Input: part model. Units: mm. Frame: model coordinates. A direction names the side the tool comes from. Round coordinates to 2 decimals unless told otherwise and drop trailing zeros. Loops run counter-clockwise (first coordinate to the right, second up) from the corner with the lowest first, then second, coordinate; pieces in that order, holes last. Notation, with made-up numbers: (32, 60.25) -> (44, 60.25) arc R21 ccw to (44, 69.25) -> close; hole circle Ø8 at (-21.5, 31.25). An arc over 180 degrees is marked (long way). Answer as a JSON object with one key per item and string values. Group by question number.
Item 1: Section query B-B on y = 15. Return loops of the section in (x, z) (3 decimals), and give its area (3 significant figures).
Item 2: Set-up query: faces 1 (the flat face through (6.35, 12, 2)), 2 (the flat face through (6, 3, -107.95)). Return all of +Z, -Z, +X, -X, +Y, -Y with unobstructed straight access to the full face (end or side cutting, diameter ignored); none if empty.
Item 3: Pin query (flat end, axial travel): pin 1 (2.5 mm diameter, centred on x = -0.29, z = -95.25, fed in from +Y); pin 2 (4.5 mm diameter, centred on x = -0.29, z = 95.25, fed in from +Y) (3 decimals); pin 3 (10 mm diameter, centred on y = 14.5, z = 49, fed in from -X). Return the tip coordinate at first contact, or that it passes through.
Item 4: Material intervals for line 1 (X direction, y = 1.5, z = -95.25) (3 decimals); line 2 (Y direction, x = -0.5, z = -71.5) (3 decimals); line 3 (X direction, y = 6.5, z = -58.5) (3 decimals), sorted ascending. Write a range as [from, to].
from build123d import *

# Parameters (mm, degrees)
BOSS_EXTRUDE1_DEPTH   = 107.95
F_6_32_TAPPED_HOLE1_D = 2.7051


with BuildPart() as part:
    # Sketch2 → Boss-Extrude1 (new, symmetric)
    with BuildSketch(Plane.XY):
        with BuildLine():
            Line((-9.525, 0), (9.525, 0))
            Line((9.525, 0), (9.525, 19.05))
            Line((9.525, 19.05), (7.9375, 19.05))
            ThreePointArc((7.9375, 19.05), (6.814967985, 18.585032015), (6.35, 17.4625))
            Line((6.35, 17.4625), (6.35, 6.35))
            ThreePointArc((6.35, 6.35), (5.42006403, 4.10493597), (3.175, 3.175))
            Line((3.175, 3.175), (-7.9375, 3.175))
            ThreePointArc((-7.9375, 3.175), (-9.060032015, 2.710032015), (-9.525, 1.5875))
            Line((-9.525, 1.5875), (-9.525, 0))
        make_face()
    extrude(amount=BOSS_EXTRUDE1_DEPTH, both=True)

    # #6-32 Tapped Hole1 (through all)
    with Locations(Plane(origin=(0, 3.175, 0), x_dir=(1, 0, 0), z_dir=(0, 1, 0))):
        with Locations((-0.2937383, -95.25), (-0.2937383, 95.25)):
            Hole(F_6_32_TAPPED_HOLE1_D / 2)


solid = part.part
Solved:
{
 "1": {"outline": "(6.35, -107.95) -> (9.525, -107.95) -> (9.525, 107.95) -> (6.35, 107.95) -> close", "area": "685 mm²"},
 "2": {"face 1": "+Z, -Z, -X, +Y", "face 2": "-Z, +X, -X, +Y, -Y"},
 "3": {"pin 1": "through", "pin 2": "y = 3.175", "pin 3": "x = 6.35"},
 "4": {"line 1": "[-9.525, -1.646], [1.059, 9.525]", "line 2": "[0, 3.175]", "line 3": "[6.35, 9.525]"}
}
